The listing builds one solid part. Answer for the finished solid, in the listing's coordinates (mm). A direction names the side the tool comes from. Give positions to 0.01 mm unless a question says otherwise; leave off trailing zeros. Order: outer loops, then holes, each group sorted by start corner. A loop starts at its lowest first (then second) coordinate and runs counter-clockwise, first axis right, second up. Notation, with made-up numbers: (67.5, 25.25) - (110.5, 25.25) arc R24 cw to (110.5, 57.25) - close; hole circle Ø1 at (-7.75, 56). An arc over 180 degrees is marked (long way). Use CSV: the item, a comma, the result in double quotes.
Autodesk Inventor part; units mm, degrees
ref_plane "YZ Plane" through (0, 0, 0) normal (1, 0, 0) x (0, 1, 0)
ref_plane "XZ Plane" through (0, 0, 0) normal (0, 1, 0) x (-1, 0, 0)
ref_plane "XY Plane" through (0, 0, 0) normal (0, 0, 1) x (1, 0, 0)
sketch "Sketch1" plane through (0, 0, 0) normal (1, 0, 0) x (0, 1, 0)
  circle A0 centre (0, 0) radius 17.78
  dimension "d0" = 35.56
extrude "Extrusion1" add sketch "Sketch1" along normal blind 58.42
sketch "Sketch2" plane through (58.42, 0, 0) normal (1, 0, 0) x (0, 0, -1)
  circle A0 centre (0, 0) radius 5
  dimension "d3" = 10
extrude "Extrusion2" add sketch "Sketch2" along normal blind 15.24
sketch "Sketch3" plane through (0, 0, 0) normal (-1, 0, 0) x (0, 0, 1)
  line L0 (0, 0) -> (-10, 0)
  line L1 (0, 0) -> (10, 0)
  line L2 (10, 2.6452) -> (12, 2.6452)
  line L3 (12, 2.6452) -> (12, -2.3548)
  line L4 (12, -2.3548) -> (10, -2.3548)
  line L5 (10, -2.3548) -> (10, 2.6452)
  line L6 (-10.4235, 2.6452) -> (-12.4235, 2.6452)
  line L7 (-12.4235, 2.6452) -> (-12.4235, -2.3548)
  line L8 (-12.4235, -2.3548) -> (-10.4235, -2.3548)
  line L9 (-10.4235, -2.3548) -> (-10.4235, 2.6452)
  dimension "d6" = 10
  dimension "d7" = 10
  dimension "d8" = 2
  dimension "d9" = 2
  dimension "d10" = 5
extrude "Extrusion3" add sketch "Sketch3" along normal blind 5
properties part number "Motor"
Item 1: The part is cut by section D-D (y = 4). Give the vertices of the cut face in (x, z), and give its area (3 significant figures).
Taken from the geometry:
outline,"(0, -17.32) - (58.42, -17.32) - (58.42, -3) - (73.66, -3) - (73.66, 3) - (58.42, 3) - (58.42, 17.32) - (0, 17.32) - close"
area,"2,120 mm^2"
Item 2: The part is cut by section C-C (x = 68.5). Give the vertices of the cut face in (y, z).
Taken from the geometry:
outline,"circle Ø10 at (0, 0)"
Item 3: Find the intervals of material crossed by line 1 along X through (y, z) = (-8.5, 5.5); line 2 along X through (y, z) = (0, 4); line 3 along Y through (x, z) = (30.5, 8), in increasing order.
Taken from the geometry:
line 1,"0 to 58.42"
line 2,"0 to 73.66"
line 3,"-15.88 to 15.88"
Item 4: Each of these flat-tipped pins is pushed along its axis until it touches: pin 1 (10.5 mm diameter, centred on y = 7.5, z = -2.5, fed in from -X); pin 2 (5.5 mm diameter, centred on x = -2, y = 0.5, fed in from +Z); pin 3 (1.6 mm diameter, centred on x = -1.5, z = -11, fed in from +Y); pin 4 (2.5 mm diameter, centred on x = -3, y = -0.5, fed in from -Z). Where does it stop, or does it pass through?
Taken from the geometry:
pin 1,"x = 0"
pin 2,"z = 17.78"
pin 3,"y = 2.65"
pin 4,"z = -12.42"
Item 5: The mould has two halves that part along Z. Classify faces 5 (the face through (-2, 0, -10.424)), 6 (the face through (-2, -2.355, 11)), 7 (the face through (-2, 0, 12)): +Z half, -Z half, draft (parallel to the pull), parting line (faces both ways), or undercut.
Taken from the geometry:
face 5,"undercut"
face 6,"draft"
face 7,"+Z half"
Item 6: The part is cut by section A-A (z = 0). Give the vertices of the cut face in (x, y).
Taken from the geometry:
outline,"(0, -17.78) - (58.42, -17.78) - (58.42, -5) - (73.66, -5) - (73.66, 5) - (58.42, 5) - (58.42, 17.78) - (0, 17.78) - close"
Item 7: The part is cut by section B-B (y = 0). Give the vertices of the cut face in (x, z), and give its area (3 significant figures).
Taken from the geometry:
outline,"(-5, -12.42) - (0, -12.42) - (0, -17.78) - (58.42, -17.78) - (58.42, -5) - (73.66, -5) - (73.66, 5) - (58.42, 5) - (58.42, 17.78) - (0, 17.78) - (0, 12) - (-5, 12) - (-5, 10) - (0, 10) - (0, -10.42) - (-5, -10.42) - close"
area,"2,250 mm^2"
Item 8: Which of the six approach directions +Z, -Z, +X, -X, +Y, -Y give full straight-line access (tool end or side, diameter ignored) to faces 1 (the face through (-2, 0, -12.424)), 2 (the face through (-2, -2.355, -11)), 3 (the face through (-2, 0, 10)), 4 (the face through (65.93, 4.88, 1.08))?
Taken from the geometry:
face 1,"-Z, -X, +Y, -Y"
face 2,"+Z, -Z, -X, -Y"
face 3,"-X, +Y, -Y"
face 4,"+X"
